```python
from build123d import *

# Parameters (mm, degrees)
SKETCH_1_R          = 1.5
EXTRUDE_1_DEPTH     = 5
SKETCH_4_W          = 40.7
SKETCH_4_H          = 19.9
CUT_EXTRUDE_1_DEPTH = 361.251648157
SKETCH_6_W          = 5
SKETCH_6_H          = 10
CUT_EXTRUDE_2_DEPTH = 361.251648157
SKETCH_7_R          = 2
CUT_EXTRUDE_3_DEPTH = 361.251648157


with BuildPart() as part:
    # 스케치1 → 보스-돌출1 (new body)
    with BuildSketch(Plane.XY):
        with BuildLine():
            Line((0, -12.5), (360, -12.5))
            Line((360, -12.5), (360, 12.5))
            Line((360, 12.5), (0, 12.5))
            ThreePointArc((0, 12.5), (-12.5, 0), (0, -12.5))
        make_face()
        with Locations((0, 7.25)):
            Circle(SKETCH_1_R, mode=Mode.SUBTRACT)
        with Locations((7.25, 0)):
            Circle(SKETCH_1_R, mode=Mode.SUBTRACT)
        with Locations((0, -7.25)):
            Circle(SKETCH_1_R, mode=Mode.SUBTRACT)
        with Locations((-7.25, 0)):
            Circle(SKETCH_1_R, mode=Mode.SUBTRACT)
    extrude(amount=EXTRUDE_1_DEPTH)

    # 스케치4 → 컷-돌출1 (cut, through all)
    with BuildSketch(Plane.XY.offset(5)):
        with Locations((330.65, 0)):
            Rectangle(SKETCH_4_W, SKETCH_4_H)
    extrude(amount=-CUT_EXTRUDE_1_DEPTH, mode=Mode.SUBTRACT)

    # 스케치6 → 컷-돌출2 (cut, through all)
    with BuildSketch(Plane.XY.offset(5)):
        with Locations((82.5, 0)):
            Rectangle(SKETCH_6_W, SKETCH_6_H)
        with Locations((202.5, 0)):
            Rectangle(SKETCH_6_W, SKETCH_6_H)
        with Locations((157.5, 0)):
            Rectangle(SKETCH_6_W, SKETCH_6_H)
        with Locations((277.5, 0)):
            Rectangle(SKETCH_6_W, SKETCH_6_H)
    extrude(amount=-CUT_EXTRUDE_2_DEPTH, mode=Mode.SUBTRACT)

    # 스케치7 → 컷-돌출3 (cut, through all)
    with BuildSketch(Plane.XY.offset(5)):
        with Locations((355, 5)):
            Circle(SKETCH_7_R)
        with Locations(Location((355, -5, 0), (0, 0, 180))):
            Circle(SKETCH_7_R)
        with Locations(Location((306.3, 5, 0), (0, 0, 180))):
            Circle(SKETCH_7_R)
        with Locations((306.3, -5)):
            Circle(SKETCH_7_R)
    extrude(amount=-CUT_EXTRUDE_3_DEPTH, mode=Mode.SUBTRACT)


solid = part.part
```
Geometry check sheet. Reference: the model listing, model coordinates, mm. Round coordinates to 2 decimals unless told otherwise and drop trailing zeros. Return JSON: item names as keys, results as strings. Group by question number.
(1) Scan lines: line 1 along Y through (x, z) = (355, 3.5); line 2 along Y through (x, z) = (0, 1.3); line 3 along Y through (x, z) = (81.5, 2.95). Record each from-to range of solid material in increasing order. Write a range as [from, to].
(2) Go/stop test with flat-tipped pins: pin 1 (3 mm diameter, centred on x = 208.5, y = 0, fed in from -Z); pin 2 (2.5 mm diameter, centred on y = 2, z = 3.5, fed in from -X); pin 3 (3 mm diameter, centred on y = -3, z = 2.5, fed in from -X). Record where each tip stops, or that it passes through.
(3) Section check A-A, the plane z = 4.25. Give the number of separate pieces and of enclosed holes in the cut face, and give its area (3 significant figures).
Data:
{
 "1": {"line 1": "[-12.5, -7], [-3, 3], [7, 12.5]", "line 2": "[-12.5, -8.75], [-5.75, 5.75], [8.75, 12.5]", "line 3": "[-12.5, -5], [5, 12.5]"},
 "2": {"pin 1": "z = 0", "pin 2": "x = -12.48", "pin 3": "x = -12.41"},
 "3": {"separate pieces": "1", "enclosed holes": "13", "area": "8,160 mm²"}
}
